```python
from build123d import *

# Parameters (mm, degrees)
BOSS_EXTRUDE1_DEPTH = 59.85
SKETCH2_R           = 17.3
BOSS_EXTRUDE2_DEPTH = 1.5
SKETCH3_R           = 15.13
SKETCH3_R_2         = 12.13
BOSS_EXTRUDE3_DEPTH = 4.5


with BuildPart() as part:
    # Sketch1 → Boss-Extrude1 (new, symmetric)
    with BuildSketch(Plane(origin=(0, 0, 0), x_dir=(1, 0, 0), z_dir=(0, 1, 0))):
        Polygon((-0.75, 0.75), (-17.15, 0.75), (-17.15, -0.75), (-0.75, -0.75), (-0.75, -17.15), (0.75, -17.15), (0.75, -0.75), (17.15, -0.75), (17.15, 0.75), (0.75, 0.75), (0.75, 17.15), (-0.75, 17.15), align=None)
    extrude(amount=BOSS_EXTRUDE1_DEPTH, both=True)

    # Sketch2 → Boss-Extrude2 (add)
    with BuildSketch(Plane(origin=(0, 59.85, 0), x_dir=(1, 0, 0), z_dir=(0, 1, 0))):
        with Locations(Location((0, 0, 0), (0, 0, 270))):
            Circle(SKETCH2_R)
    boss_extrude2 = extrude(amount=BOSS_EXTRUDE2_DEPTH)

    # Mirror1: Boss-Extrude2 across plane
    add(boss_extrude2.mirror(Plane.ZX))

    # Sketch3 → Boss-Extrude3 (add, symmetric)
    with BuildSketch(Plane.XY):
        with Locations((0, 75.35)):
            Circle(SKETCH3_R)
        with Locations((0, 75.35)):
            Circle(SKETCH3_R_2, mode=Mode.SUBTRACT)
    extrude(amount=BOSS_EXTRUDE3_DEPTH, both=True)

    # Sketch4 → Revolve1 (revolve)
    with BuildSketch(Plane(origin=(0, 0, 0), x_dir=(0, 0, -1), z_dir=(1, 0, 0))):
        Polygon((-5.95, -61.35), (-5.95, -65.35), (-14.15, -65.35), (-14.15, -66.85), (-13.15, -67.85), (0, -67.85), (0, -61.35), align=None)
    revolve(axis=Axis((0, -54.373859454, 0), (0, -1, 0)))


solid = part.part
```
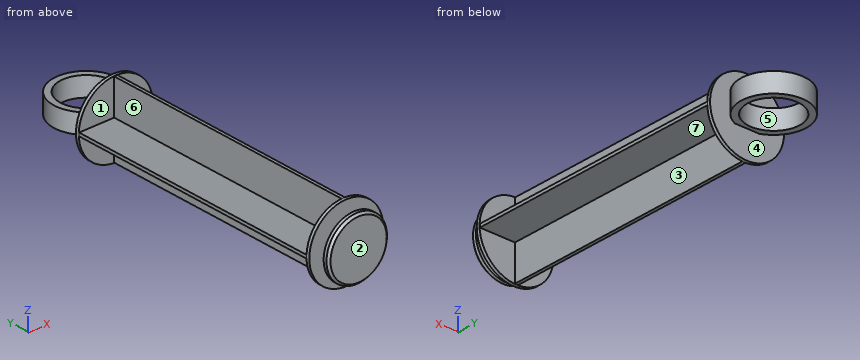
Geometry check sheet. Reference: the model listing, model coordinates, mm. Face numbers are marked on the shaded views. A direction names the side the tool comes from. Round coordinates to 2 decimals unless told otherwise and drop trailing zeros. Loops run counter-clockwise (first coordinate to the right, second up) from the corner with the lowest first, then second, coordinate; pieces in that order, holes last. Notation, with made-up numbers: (24, 80.5) - (32, 80.5) arc R10 ccw to (32, 93.5) - close; hole circle Ø10 at (-28.75, -38). An arc over 180 degrees is marked (long way). Write item = value, one per line. Start each with the question number.
1. Set-up check for the marked faces 4, 5, 6 and 7: record each of +Z, -Z, +X, -X, +Y, -Y from which the full face is reachable in a straight line by a thin tool's end or side.
2. Section check B-B on y = 38. Enter the section's corners in (x, z), then the cut area to 3 significant figures.
3. Section check A-A on y = 75.35. Enter the section's corners in (x, z).
4. Depth check by flat-ended pin: pin 1 (18 mm diameter, centred on y = 30, z = 7, fed in from -X); pin 2 (19.5 mm diameter, centred on x = 0, y = 75.35, fed in from -Z); pin 3 (1 mm diameter, centred on x = 12.5, y = -12.5, fed in from -Z); pin 4 (4 mm diameter, centred on x = 5, z = 5.5, fed in from +Y). Enter the tip coordinate at first touch or a pass-through.
5. Thickness scan on line 1 (Y direction, x = 7.5, z = -13); line 2 (Y direction, x = -4, z = -7.5); line 3 (X direction, y = 75, z = 1). Record the ranges inside material, lowest first.
6. Mould release check, pull along Y, two halves, no side actions. Record for the marked faces 1, 2 and 3: released by +Y, released by -Y, zero draft, split by the parting line, or undercut.
Working result:
q1.face_4 = none
q1.face_5 = +Z, -Z
q1.face_6 = +Z, -X
q1.face_7 = -Z, +X
q2.outline = (-17.15, -0.75) - (-0.75, -0.75) - (-0.75, -17.15) - (0.75, -17.15) - (0.75, -0.75) - (17.15, -0.75) - (17.15, 0.75) - (0.75, 0.75) - (0.75, 17.15) - (-0.75, 17.15) - (-0.75, 0.75) - (-17.15, 0.75) - close
q2.area = 101 mm^2
q3.outline = (-15.13, -4.5) - (-12.13, -4.5) - (-12.13, 4.5) - (-15.13, 4.5) - close; (12.13, -4.5) - (15.13, -4.5) - (15.13, 4.5) - (12.13, 4.5) - close
q4.pin_1 = -17.15
q4.pin_2 = through
q4.pin_3 = -0.75
q4.pin_4 = 90.12
q5.line_1 = -61.35 to -59.85, 59.85 to 61.35
q5.line_2 = -67.85 to -65.35, -61.35 to -59.85, 59.85 to 61.35
q5.line_3 = -15.13 to -12.12, 12.12 to 15.13
q6.face_1 = undercut
q6.face_2 = released by -Y
q6.face_3 = undercut
